Read the model definition and answer for the solid it produces. Units are mm, in the model's axes. A direction names the side the tool comes from. Give positions to 0.01 mm unless a question says otherwise; leave off trailing zeros. Loops run counter-clockwise (first coordinate to the right, second up) from the corner with the lowest first, then second, coordinate; pieces in that order, holes last.
(1) Straight lines are drawn through the part: probe 1 along Y at (x, z) = (63.81, -9.5); probe 2 along X at (y, z) = (2.25, -10); probe 3 along Y at (x, z) = (76, 11). For each, find the intervals that lie inside material, in ascending order.
(2) Determine the mould class of faces 5 (the face through (38, 30, 23)), 6 (the face through (0, 10, 14)), 7 (the face through (16, 21, -12)) for opening direction Z: pulls with the +Z half, pulls with the -Z half, needs draft (parallel to the pull), parting line crosses it, or undercut.
(3) Find section D-D, the plane y = 31. Write down the section's boundary in (x, z).
(4) Find section B-B, the plane x = 75. Write down the section's boundary in (y, z).
(5) Find section C-C, the plane y = 1. Write down the section's boundary in (x, z).
(6) Which of the six approach directions +Z, -Z, +X, -X, +Y, -Y give full straight-line access (tool end or side, diameter ignored) to faces 1 (the face through (16, 16, 0)), 2 (the face through (10, 26.12, 6)), 3 (the face through (64, 16, 0)), 4 (the face through (8, 6.12, -11))?
(7) Each of these flat-tipped pins is pushed along its axis until it touches: P1, Ø9, axis at x = 7.5, y = 14.5, coming from the +Z side; P2, Ø10.5, axis at x = 6, z = -7, coming from the +Y side; P3, Ø6, axis at x = 46, z = 1.5, coming from the -Y side; P4, Ø2.5, axis at x = 63.81, y = 10.946, coming from the +Z side. Where does it stop, or does it pass through?
(8) Find section A-A, the plane z = -15. Write down the section's boundary in (x, y), then the cut area to 3 significant figures.
```python
from build123d import *

# Parameters (mm, degrees)
SKETCH1_W           = 80
SKETCH1_H           = 20
BOSS_EXTRUDE1_DEPTH = 6.12
SKETCH14_R          = 2
CUT_EXTRUDE7_DEPTH  = 22.92
SKETCH2_W           = 7
SKETCH2_H           = 20
BOSS_EXTRUDE2_DEPTH = 20
SKETCH3_W           = 80
SKETCH3_H           = 6.12
BOSS_EXTRUDE3_DEPTH = 35
SKETCH5_R           = 21
BOSS_EXTRUDE4_DEPTH = 12
SKETCH4_R           = 16
CUT_EXTRUDE1_DEPTH  = 12
SKETCH7_R           = 1.5
CUT_EXTRUDE2_DEPTH  = 12
CUT_EXTRUDE4_DEPTH  = 10
SKETCH15_W          = 40.4
SKETCH15_H          = 20
CUT_EXTRUDE8_DEPTH  = 20
SKETCH16_W          = 13
SKETCH16_H          = 26
BOSS_EXTRUDE6_DEPTH = 20
CHAMFER1_SIZE       = 6.5


with BuildPart() as part:
    # Sketch1 → Boss-Extrude1 (new body)
    with BuildSketch(Plane(origin=(0, 0, 0), x_dir=(1, 0, 0), z_dir=(0, 1, 0))):
        with Locations((40, 10)):
            Rectangle(SKETCH1_W, SKETCH1_H)
    extrude(amount=BOSS_EXTRUDE1_DEPTH)

    # Sketch14 → Cut-Extrude7 (cut)
    with BuildSketch(Plane(origin=(0, 6.12, 0), x_dir=(1, 0, 0), z_dir=(0, 1, 0))):
        with Locations(Location((75, 10, 0), (0, 0, 270))):
            Circle(SKETCH14_R)
        with Locations(Location((5, 10, 0), (0, 0, 270))):
            Circle(SKETCH14_R)
    extrude(amount=-CUT_EXTRUDE7_DEPTH, mode=Mode.SUBTRACT)

    # Sketch2 → Boss-Extrude2 (add)
    with BuildSketch(Plane(origin=(0, 6.12, 0), x_dir=(1, 0, 0), z_dir=(0, 1, 0))):
        with Locations((16.5, 10)):
            Rectangle(SKETCH2_W, SKETCH2_H)
        with Locations((63.5, 10)):
            Rectangle(SKETCH2_W, SKETCH2_H)
    extrude(amount=BOSS_EXTRUDE2_DEPTH)

    # Sketch3 → Boss-Extrude3 (add)
    with BuildSketch(Plane.XY):
        with Locations((40, 3.06)):
            Rectangle(SKETCH3_W, SKETCH3_H)
    extrude(amount=BOSS_EXTRUDE3_DEPTH)

    # Sketch5 → Boss-Extrude4 (add)
    with BuildSketch(Plane.XY.offset(35)):
        with Locations((29.774, 16.026)):
            Circle(SKETCH5_R)
    extrude(amount=-BOSS_EXTRUDE4_DEPTH)

    # Sketch4 → Cut-Extrude1 (cut)
    with BuildSketch(Plane.XY.offset(35)):
        with Locations((29.774, 16.026)):
            Circle(SKETCH4_R)
    extrude(amount=-CUT_EXTRUDE1_DEPTH, mode=Mode.SUBTRACT)

    # Sketch7 → Cut-Extrude2 (cut)
    with BuildSketch(Plane.XY):
        with Locations((16.312, 21.106)):
            Circle(SKETCH7_R)
        with Locations((16.312, 10.946)):
            Circle(SKETCH7_R)
        with Locations((63.81, 10.946)):
            Circle(SKETCH7_R)
        with Locations((63.81, 21.106)):
            Circle(SKETCH7_R)
    extrude(amount=-CUT_EXTRUDE2_DEPTH, mode=Mode.SUBTRACT)

    # Sketch9 → Cut-Extrude4 (cut)
    with BuildSketch(Plane(origin=(0, 6.12, 0), x_dir=(1, 0, 0), z_dir=(0, 1, 0))):
        Polygon((80, -19), (64, -35), (80, -35), align=None)
    extrude(amount=-CUT_EXTRUDE4_DEPTH, mode=Mode.SUBTRACT)

    # Sketch15 → Cut-Extrude8 (cut)
    with BuildSketch(Plane(origin=(0, 26.12, 0), x_dir=(1, 0, 0), z_dir=(0, 1, 0))):
        with Locations((40, 10)):
            Rectangle(SKETCH15_W, SKETCH15_H)
    extrude(amount=-CUT_EXTRUDE8_DEPTH, mode=Mode.SUBTRACT)

    # Sketch16 → Boss-Extrude6 (add)
    with BuildSketch(Plane(origin=(0, 6.12, 0), x_dir=(1, 0, 0), z_dir=(0, 1, 0))):
        with Locations((6.5, -10)):
            Rectangle(SKETCH16_W, SKETCH16_H)
    extrude(amount=BOSS_EXTRUDE6_DEPTH)

    # Chamfer1
    chamfer1_edges = [part.edges().sort_by_distance(p)[0] for p in [
        (13, 16.12, -3),
    ]]
    chamfer(chamfer1_edges, length=CHAMFER1_SIZE)
    chamfer1_2_edges = [part.edges().sort_by_distance(p)[0] for p in [
        (0, 16.12, -3),
    ]]
    chamfer(chamfer1_2_edges, length=CHAMFER1_SIZE - 0.0001)  # a hair under: the kernel refuses the full size


solid = part.part
```
Entries:
1. probe 1: y = 0 to 9.45, 12.45 to 19.61, 22.61 to 26.12
1. probe 2: x = 0 to 3, 7 to 73, 77 to 80
1. probe 3: y = 0 to 6.12
2. face 5: undercut
2. face 6: needs draft
2. face 7: pulls with the +Z half
3. outline: (15.05, 23) - (24.14, 23) - (24.14, 35) - (15.05, 35) - close; (35.41, 23) - (44.5, 23) - (44.5, 35) - (35.41, 35) - close
4. outline: (0, -20) - (6.12, -20) - (6.12, -12) - (0, -12) - close; (0, -8) - (6.12, -8) - (6.12, 24) - (0, 24) - close
5. outline: (0, -20) - (80, -20) - (80, 19) - (64, 35) - (35.27, 35) - (35.27, 23) - (24.28, 23) - (24.28, 35) - (0, 35) - close; hole circle Ø4 at (5, -10); hole circle Ø4 at (75, -10)
6. face 1: +X, +Y
6. face 2: -Z, +X, -X, +Y
6. face 3: +Z, +X, +Y
6. face 4: -Z, -X, +Y
7. P1: stops at z = 35
7. P2: stops at y = 26.12
7. P3: stops at y = 0
7. P4: stops at z = -12
8. outline: (0, 0) - (80, 0) - (80, 6.12) - (67, 6.12) - (67, 26.12) - (60.2, 26.12) - (60.2, 6.12) - (19.8, 6.12) - (19.8, 26.12) - (13, 26.12) - (13, 6.12) - (0, 6.12) - close
8. area: 762 mm2
